Geometry check sheet. Reference: the model listing, model coordinates, mm. A direction names the side the tool comes from. Round coordinates to 2 decimals unless told otherwise and drop trailing zeros. Loops run counter-clockwise (first coordinate to the right, second up) from the corner with the lowest first, then second, coordinate; pieces in that order, holes last. Notation, with made-up numbers: (0, 76.5) - (12, 76.5) arc R24 ccw to (12, 108.5) - close; hole circle Ø1 at (37, 57). An arc over 180 degrees is marked (long way). Write item = value, one per line.
```python
from build123d import *

# Parameters (mm, degrees)
SKETCH2_W                    = 127
SKETCH2_H                    = 25.4
BASE_FLANGE1_DEPTH           = 3.175
EDGE_FLANGE1_STRIP_W         = 14.7
EDGE_FLANGE1_STRIP_H         = 3.175
EDGE_FLANGE1_STRIP_CUT_DEPTH = 25.4
EDGE_FLANGE1_DEPTH           = 25.4
CUT_EXTRUDE1_REACH           = 144.875
SKETCH10_R                   = 5.08


# Sheet-metal steps are written as plain solids
with BuildPart() as part:
    # Sketch2 → Base-Flange1 (new body)
    with BuildSketch(Plane(origin=(0, 0, 0), x_dir=(1, 0, 0), z_dir=(0, 1, 0))):
        with Locations((63.5, 12.7)):
            Rectangle(SKETCH2_W, SKETCH2_H)
    extrude(amount=-BASE_FLANGE1_DEPTH)

    # Edge-Flange1 strip (across the edge) → Edge-Flange1 strip cut (cut)
    with BuildSketch(Plane(origin=(127, 0, 0), x_dir=(-1, 0, 0), z_dir=(0, 0, -1))):
        with Locations((-3.175, -1.5875)):
            Rectangle(EDGE_FLANGE1_STRIP_W, EDGE_FLANGE1_STRIP_H)
    extrude(amount=EDGE_FLANGE1_STRIP_CUT_DEPTH, mode=Mode.SUBTRACT)

    # Edge-Flange1 section (across the edge) → Edge-Flange1 (add)
    with BuildSketch(Plane(origin=(127, 0, 0), x_dir=(-1, 0, 0), z_dir=(0, 0, -1))):
        with BuildLine():
            Line((0, 1), (0, 60.325))
            Line((0, 60.325), (3.175, 60.325))
            Line((3.175, 60.325), (3.175, 1))
            ThreePointArc((3.175, 1), (3.467893219, 0.292893219), (4.175, 0))
            Line((4.175, 0), (4.175, -3.175))
            ThreePointArc((4.175, -3.175), (1.222829189, -1.952170811), (0, 1))
        make_face()
    extrude(amount=EDGE_FLANGE1_DEPTH)

    # Sketch10 → Cut-Extrude1 (cut, up to next)
    with BuildSketch(Plane(origin=(127, 0, 0), x_dir=(0, 0, -1), z_dir=(1, 0, 0)), mode=Mode.PRIVATE) as cut_extrude1_sk1:
        with Locations(Location((12.7, 36.5125, 0), (0, 0, 90))):
            Circle(SKETCH10_R)
    cut_extrude1_tool1 = extrude(cut_extrude1_sk1.sketch, amount=-CUT_EXTRUDE1_REACH, mode=Mode.PRIVATE) & part.part
    add(cut_extrude1_tool1.solids().sort_by_distance((127, 36.5125, -12.7))[0], mode=Mode.SUBTRACT)


solid = part.part
```
(1) Set-up check for faces 1 (the flat face through (125, 60.325, -13)), 2 (the flat face through (61, 0, -13)): record each of +Z, -Z, +X, -X, +Y, -Y from which the full face is reachable in a straight line by a thin tool's end or side.
Answers follow:
face_1 = +Z, -Z, +X, -X, +Y
face_2 = +Z, -Z, -X, +Y
(2) Scan lines: L1, parallel to Y at x = 23, z = -4 (3 decimals); L2, parallel to X at y = 31.5, z = -14.5 (3 decimals). Record each from-to range of solid material in increasing order. Write a range as [from, to].
Answers follow:
L1 = [-3.175, 0]
L2 = [123.825, 127]
(3) Section check B-B (y = 39). Enter the section's corners in (x, z) (3 decimals), then the cut area to 3 significant figures.
Answers follow:
outline = (123.825, -25.4) - (127, -25.4) - (127, -17.129) - (123.825, -17.129) - close; (123.825, -8.271) - (127, -8.271) - (127, 0) - (123.825, 0) - close
area = 52.5 mm²
(4) Section check D-D (x = 61.5). Enter the section's corners in (y, z) (3 decimals), then the cut area to 3 significant figures.
Answers follow:
outline = (-3.175, -25.4) - (0, -25.4) - (0, 0) - (-3.175, 0) - close
area = 80.6 mm²
(5) Section check C-C (z = -21). Enter the section's corners in (x, y) (3 decimals).
Answers follow:
outline = (0, -3.175) - (122.825, -3.175) arc R4.175 ccw to (127, 1) - (127, 60.325) - (123.825, 60.325) - (123.825, 1) arc R1 cw to (122.825, 0) - (0, 0) - close
(6) Gauge pin test, flat ends, axial feed: pin 1 (3 mm diameter, centred on y = 39, z = -14.5, fed in from -X); pin 2 (12 mm diameter, centred on y = 45.5, z = -17, fed in from -X) (3 decimals); pin 3 (7.5 mm diameter, centred on x = 61, z = -10, fed in from +Y). Record the tip position at first contact, or that the pin passes through.
Answers follow:
pin_1 = through
pin_2 = 123.825
pin_3 = 0
(7) Mould release check, pull along Z, two halves, no side actions. Record for faces 3 (the cylindrical face through (125.43, 32.48, -15.79)), 4 (the flat face through (91, -2, -25.4)), 5 (the flat face through (123.825, 31, -13)), 6 (the flat face through (91, -2, 0)): pulls with the +Z half, pulls with the -Z half, needs draft (parallel to the pull), parting line crosses it, or undercut.
Answers follow:
face_3 = undercut
face_4 = pulls with the -Z half
face_5 = needs draft
face_6 = pulls with the +Z half
